from build123d import *

# Parameters (mm, degrees)
F1_DEPTH = 2
F3_DEPTH = 3
F4_R     = 5
F5_R     = 5
F6_W     = 10.114867
F6_H     = 22.403944
F6_W_2   = 7.454773
F6_H_2   = 19.985135
F6_W_3   = 0.818297
F6_H_3   = 2.934326
F7_DEPTH = 0.5


with BuildPart() as f1:
    # F0 (on Top) → F1 (new body)
    with BuildSketch(Plane.XY):
        with BuildLine():
            Line((0, 63), (0, 0))
            Line((0, 0), (15, 0))
            Line((15, 0), (25, 10))
            Line((25, 10), (25, 43))
            Line((25, 43), (15.5, 43))
            ThreePointArc((15.5, 43), (12.93934, 41.93934), (14, 44.5))
            Line((14, 44.5), (14, 63))
            Line((14, 63), (0, 63))
        make_face()
    extrude(amount=F1_DEPTH)

    # F2 (on face) → F3 (join)
    with BuildSketch(Plane(origin=(0, 0, 0), x_dir=(1, 0, 0), z_dir=(0, 0, -1))):
        Polygon((15, 0), (0, 0), (0, -3), (18, -3), align=None)
        Polygon((25, -43), (25, -10), (22, -7), (22, -43), align=None)
    extrude(amount=F3_DEPTH)

    # F4
    f4_edges = [f1.edges().sort_by_distance(p)[0] for p in [
        (14, 44.5, 1),
        (15.5, 43, 1),
    ]]
    fillet(f4_edges, radius=F4_R)

    # F5
    f5_edges = [f1.edges().sort_by_distance(p)[0] for p in [
        (0, 63, 1),
        (0, 0, -0.5),
        (15, 0, -0.5),
        (25, 10, -0.5),
    ]]
    fillet(f5_edges, radius=F5_R)

    # F6 (on face) → F7 (cut)
    with BuildSketch(Plane.XY.offset(2)):
        with Locations((14.416239, 28.307009)):
            Rectangle(F6_W, F6_H)
        with Locations((14.355088, 28.207892)):
            Rectangle(F6_W_2, F6_H_2, mode=Mode.SUBTRACT)
        Polygon((5.570976, 25.942754), (3.440016, 24.428651), (5.570976, 22.914547), (5.570976, 23.867872), (8.150558, 23.867872), (8.09448, 24.428651), (8.150558, 24.98943), (5.570976, 24.98943), align=None)
        Polygon((13.157818, 13.575147), (14.671921, 11.444188), (16.186024, 13.575147), (15.2327, 13.575147), (15.2327, 16.15473), (14.671921, 16.098652), (14.111142, 16.15473), (14.111142, 13.575147), align=None)
        with BuildLine():
            Line((11.334654, 19.87192), (11.334654, 18.880593))
            Line((11.334654, 18.880593), (12.444939, 18.880593))
            Line((12.444939, 18.880593), (12.444939, 19.760527))
            ThreePointArc((12.444939, 19.760527), (12.477566, 19.839294), (12.556333, 19.87192))
            Line((12.556333, 19.87192), (13.555225, 19.87192))
            Line((13.555225, 19.87192), (13.555225, 20.791506))
            ThreePointArc((13.555225, 20.791506), (13.587851, 20.870274), (13.666619, 20.9029))
            Line((13.666619, 20.9029), (14.625858, 20.9029))
            Line((14.625858, 20.9029), (14.625858, 22.092491))
            Line((14.625858, 22.092491), (13.555225, 22.092491))
            Line((13.555225, 22.092491), (13.555225, 21.014294))
            ThreePointArc((13.555225, 21.014294), (13.522599, 20.935526), (13.443831, 20.9029))
            Line((13.443831, 20.9029), (12.556333, 20.9029))
            ThreePointArc((12.556333, 20.9029), (12.477566, 20.935526), (12.444939, 21.014294))
            Line((12.444939, 21.014294), (12.444939, 22.568326))
            Line((12.444939, 22.568326), (14, 22.568326))
            Line((14, 22.568326), (14, 23.487912))
            ThreePointArc((14, 23.487912), (14.032626, 23.56668), (14.111394, 23.599306))
            Line((14.111394, 23.599306), (16.848227, 23.599306))
            Line((16.848227, 23.599306), (16.848227, 24.515837))
            Line((16.848227, 24.515837), (14, 24.515837))
            Line((14, 24.515837), (14, 23.7107))
            ThreePointArc((14, 23.7107), (13.967374, 23.631933), (13.888606, 23.599306))
            Line((13.888606, 23.599306), (12.444939, 23.599306))
            Line((12.444939, 23.599306), (12.444939, 24.55098))
            Line((12.444939, 24.55098), (11.334654, 24.55098))
            Line((11.334654, 24.55098), (11.334654, 22.050673))
            Line((11.334654, 22.050673), (11.334654, 20.9029))
            Line((11.334654, 20.9029), (12.333546, 20.9029))
            ThreePointArc((12.333546, 20.9029), (12.412313, 20.870274), (12.444939, 20.791506))
            Line((12.444939, 20.791506), (12.444939, 19.983314))
            ThreePointArc((12.444939, 19.983314), (12.412313, 19.904547), (12.333546, 19.87192))
            Line((12.333546, 19.87192), (11.334654, 19.87192))
        make_face()
        with Locations((16.497659, 20.506369)):
            Rectangle(F6_W_3, F6_H_3)
    extrude(amount=-F7_DEPTH, mode=Mode.SUBTRACT)


solid = f1.part
Geometry check sheet. Reference: the model listing, model coordinates, mm. A direction names the side the tool comes from. Give positions to 0.01 mm unless a question says otherwise; leave off trailing zeros. Loops run counter-clockwise (first coordinate to the right, second up) from the corner with the lowest first, then second, coordinate; pieces in that order, holes last. Notation, with made-up numbers: (39.25, 30) -> (43.25, 30) arc R12 cw to (43.25, 42) -> close; hole circle Ø7 at (-40, -26). An arc over 180 degrees is marked (long way). Answer in a Markdown table with one row per item. Add a question column.
1) Cross-section at D-D on y = 48. Record the boundary of the cut face in (x, z).
2) Material ranges on probe 1 along X at (y, z) = (33.5, -2.5); probe 2 along Z at (x, y) = (7.75, 37); probe 3 along Z at (x, y) = (16, 13.5), recorded low to high. Write a range as from..to.
3) Gauge pin test, flat end, axial feed: P1, Ø10, axis at x = 10, y = 50.5, coming from the -Z side. Record the tip position at first contact, or that the pin passes through.
4) Draft check along Y on faces 6 (the face through (10, 63, 1)), 7 (the face through (14, 28, 2)), 8 (the face through (19, 30, 1.5)), 9 (the face through (13, 23, 1.5)). Enter one of: pulls with the +Y half, pulls with the -Y half, needs draft (parallel to the pull), parting line crosses it, or undercut.
5) Cross-section at B-B on x = 8.75. Record the boundary of the cut face in (y, z).
6) Cross-section at C-C on y = 27. Record the boundary of the cut face in (x, z), and give its area (3 significant figures).
7) Set-up check for faces 1 (the face through (11, 33, 0)), 2 (the face through (9, 3, -1)), 3 (the face through (1, 61, 1)), 4 (the face through (14, 55, 1)), 5 (the face through (24.63, 10.18, -0.46)): record each of +Z, -Z, +X, -X, +Y, -Y from which the full face is reachable in a straight line by a thin tool's end or side.
8) Cross-section at A-A on z = -1.2. Record the boundary of the cut face in (x, y), and give its area (3 significant figures).
Outcome:
| question | item | result |
|---|---|---|
| 1 | outline | (0, 0) -> (14, 0) -> (14, 2) -> (0, 2) -> close |
| 2 | probe 1 | x = 22..25 |
| 2 | probe 2 | z = 0..2 |
| 2 | probe 3 | z = 0..1.5 |
| 3 | P1 | stops at z = 0 |
| 4 | face 6 | pulls with the +Y half |
| 4 | face 7 | needs draft |
| 4 | face 8 | undercut |
| 4 | face 9 | undercut |
| 5 | outline | (0, -3) -> (3, -3) -> (3, 0) -> (63, 0) -> (63, 2) -> (0, 2) -> close |
| 6 | outline | (0, 0) -> (22, 0) -> (22, -3) -> (25, -3) -> (25, 2) -> (19.47, 2) -> (19.47, 1.5) -> (18.08, 1.5) -> (18.08, 2) -> (10.63, 2) -> (10.63, 1.5) -> (9.36, 1.5) -> (9.36, 2) -> (0, 2) -> close |
| 6 | area | 57.7 mm^2 |
| 7 | face 1 | -Z, -X, +Y |
| 7 | face 2 | -Z, +X, -X, +Y |
| 7 | face 3 | +Z, -Z, -X, +Y |
| 7 | face 4 | +Z, -Z, +X, +Y |
| 7 | face 5 | +Z, -Z, +X, -Y |
| 8 | outline | (0.42, 3) arc R5 ccw to (5, 0) -> (12.93, 0) arc R5 ccw to (16.46, 1.46) -> (18, 3) -> close; (22, 7) -> (23.54, 8.54) arc R5 ccw to (25, 12.07) -> (25, 43) -> (22, 43) -> close |
| 8 | area | 147 mm^2 |
